Can you work these out from the model? Positions are in its coordinate system, mm. Give positions to 0.01 mm unless a question says otherwise; leave off trailing zeros. Order: outer loops, then holes, each group sorted by start corner. A loop starts at its lowest first (then second) coordinate and runs counter-clockwise, first axis right, second up. Notation, with made-up numbers: M -18,61.25 L 17,61.25 A6 ccw 17,65.25 Z; hole C 23.25,49.5 d4. An arc over 180 degrees is marked long. Use one line per item in the form item = value. Start each with the question number.
1. I need wall thicknesses on L1, parallel to X at y = -0.5, z = 0.45; L2, parallel to Y at x = -0.5, z = 1; L3, parallel to Y at x = 1.75, z = 0.2. Which ranges of each line are inside material? Lowest first, please.
2. I want a section at D-D, the plane x = -4. List the corners of the cut face in (y, z) for me.
3. I want a section at B-B, the plane y = -1. List the corners of the cut face in (x, z) for me, and give its area (3 significant figures).
4. We'd pull the mould along Y, two halves only. Please class faces 1 (the face through (0, 5.99, 1)), 2 (the face through (1.22, -1.28, 0.99)), 3 (the face through (6.206, 0, 1)): +Y half, -Y half, draft (parallel to the pull), parting line (faces both ways), or undercut.
5. I want a section at C-C, the plane z = 0.7. List the corners of the cut face in (x, y) for me, and give its area (3 significant figures).
6. I want a section at A-A, the plane x = 0. List the corners of the cut face in (y, z) for me, and give its area (3 significant figures).
Autodesk Inventor part; units mm, degrees
ref_plane "YZ Plane" through (0, 0, 0) normal (1, 0, 0) x (0, 1, 0)
ref_plane "XZ Plane" through (0, 0, 0) normal (0, 1, 0) x (-1, 0, 0)
ref_plane "XY Plane" through (0, 0, 0) normal (0, 0, 1) x (1, 0, 0)
sketch "washer_sketch" plane through (0, 0, 0) normal (0, 0, 1) x (1, 0, 0)
  line L0 (-5.3709, -5.3107) -> (-5.3709, 4.5904) construction
  line L1 (0.3709, -5.3107) -> (-5.3709, -5.3107) construction
  arc A0 (0.3709, -5.3107) -> (5.3709, -0.3107) centre (0.3709, -0.3107) ccw construction
  arc A1 (5.3709, -0.3107) -> (-3.0036, 4.5904) centre (-0.2505, -0.3107) ccw construction
  line L2 (-5.3709, 4.5904) -> (-3.0036, 4.5904) construction
  circle A2 centre (0.4177, -0.0104) radius 3.55 construction
  circle A3 centre (0.4177, -0.0104) radius 3.55 construction
  circle A4 centre (0.4177, -0.0104) radius 1.5
  line L3 (4.2064, 5.9896) -> (-3.3709, 5.9896)
  line L4 (-5.3709, 3.9896) -> (-5.3709, -4.0104)
  line L5 (-3.3709, -6.0104) -> (4.2064, -6.0104)
  line L6 (6.2064, -4.0104) -> (6.2064, 3.9896)
  arc A5 (6.2064, 3.9896) -> (4.2064, 5.9896) centre (4.2064, 3.9896) ccw
  arc A6 (4.2064, -6.0104) -> (6.2064, -4.0104) centre (4.2064, -4.0104) ccw
  arc A7 (-5.3709, -4.0104) -> (-3.3709, -6.0104) centre (-3.3709, -4.0104) ccw
  arc A8 (-3.3709, 5.9896) -> (-5.3709, 3.9896) centre (-3.3709, 3.9896) ccw
  point P0 (0, 0)
  point P1 (6.2064, 5.9896)
  point P2 (-5.3709, 5.9896)
  point P3 (6.2064, -6.0104)
  dimension "d0" = 12
  dimension "d1" = 11.5773
  dimension "d2" = 5.7886
  dimension "d3" = 6
  dimension "d4" = 2
extrude "washer" add sketch "washer_sketch" along normal blind 2
equation "\"d3\" = 0.5 * d0"
properties part number "mount_linear_stepper_washer_b"
Check result:
q1.L1 = -5.37 to -1, 1.84 to 6.21
q1.L2 = -6.01 to -1.2, 1.18 to 5.99
q1.L3 = -6.01 to -0.7, 0.68 to 5.99
q2.outline = M -5.91,0 L 5.89,0 L 5.89,2 L -5.91,2 Z
q3.outline = M -5.37,0 L -0.71,0 L -0.71,2 L -5.37,2 Z; M 1.54,0 L 6.21,0 L 6.21,2 L 1.54,2 Z
q3.area = 18.6 mm2
q4.face_1 = +Y half
q4.face_2 = undercut
q4.face_3 = draft
q5.outline = M -5.37,-4.01 A2 ccw -3.37,-6.01 L 4.21,-6.01 A2 ccw 6.21,-4.01 L 6.21,3.99 A2 ccw 4.21,5.99 L -3.37,5.99 A2 ccw -5.37,3.99 Z; hole C 0.42,-0.01 d3
q5.area = 128 mm2
q6.outline = M -6.01,0 L -1.45,0 L -1.45,2 L -6.01,2 Z; M 1.43,0 L 5.99,0 L 5.99,2 L 1.43,2 Z
q6.area = 18.2 mm2
